from build123d import *

# Parameters (mm, degrees)
SKETCH1_W               = 78
SKETCH1_H               = 48
BOSS_EXTRUDE1_DEPTH     = 32
CUT_EXTRUDE1_DEPTH      = 1
CUT_EXTRUDE1_DEPTH_BACK = 49
SKETCH3_OUTSIDE_W       = 69.404
SKETCH3_OUTSIDE_H       = 53.404
CUT_EXTRUDE3_DEPTH      = 1
CUT_EXTRUDE3_DEPTH_BACK = 79
FILLET1_R               = 1.5
SKETCH4_R               = 4
CUT_EXTRUDE4_DEPTH      = 1
CUT_EXTRUDE4_DEPTH_BACK = 10
CHAMFER1_SIZE           = 1.5


with BuildPart() as part:
    # Sketch1 → Boss-Extrude1 (new body)
    with BuildSketch(Plane(origin=(0, 0, 0), x_dir=(1, 0, 0), z_dir=(0, 1, 0))):
        Rectangle(SKETCH1_W, SKETCH1_H)
    extrude(amount=BOSS_EXTRUDE1_DEPTH)

    # Sketch2 → Cut-Extrude1 (cut, two sides)
    with BuildSketch(Plane.XY.offset(24)) as cut_extrude1_sk:
        Polygon((-39, 13.33), (-35.438170518, 21.33), (-35.438170518, 32), (-39, 32), align=None)
        Polygon((35.438170518, 21.33), (35.438170518, 32), (39, 32), (39, 13.33), align=None)
    extrude(amount=CUT_EXTRUDE1_DEPTH, mode=Mode.SUBTRACT)
    extrude(cut_extrude1_sk.sketch, amount=-CUT_EXTRUDE1_DEPTH_BACK, mode=Mode.SUBTRACT)

    # Sketch3 outside → Cut-Extrude3 (cut, two sides)
    with BuildSketch(Plane(origin=(39, 0, 0), x_dir=(0, 0, -1), z_dir=(1, 0, 0))) as cut_extrude3_sk:
        with Locations((0, 16)):
            Rectangle(SKETCH3_OUTSIDE_W, SKETCH3_OUTSIDE_H)
        Polygon((-24, 8), (-18, 4.535898385), (-18, 32), (0, 32), (0, 25), (1.787630389, 26.5), (3.787630389, 26.5), (5.575260778, 25), (24, 25), (24, 10.67), (-4.8, 10.67), (-4.8, 0), (-24, 0), align=None, mode=Mode.SUBTRACT)
    extrude(amount=CUT_EXTRUDE3_DEPTH, mode=Mode.SUBTRACT)
    extrude(cut_extrude3_sk.sketch, amount=-CUT_EXTRUDE3_DEPTH_BACK, mode=Mode.SUBTRACT)

    # Fillet1
    fillet1_edges = [part.edges().sort_by_distance(p)[0] for p in [
        (0, 0, 24),
        (0, 10.67, 4.8),
        (0, 4.535898385, 18),
        (0, 0, 4.8),
        (0, 10.67, -24),
    ]]
    fillet(fillet1_edges, radius=FILLET1_R)

    # Sketch4 → Cut-Extrude4 (cut, two sides)
    with BuildSketch(Plane(origin=(0, 32, 0), x_dir=(1, 0, 0), z_dir=(0, 1, 0))) as cut_extrude4_sk:
        with Locations((0, -9)):
            Circle(SKETCH4_R)
        with Locations((23.438170518, -9)):
            Circle(SKETCH4_R)
        with Locations((-23.438170518, -9)):
            Circle(SKETCH4_R)
    extrude(amount=CUT_EXTRUDE4_DEPTH, mode=Mode.SUBTRACT)
    extrude(cut_extrude4_sk.sketch, amount=-CUT_EXTRUDE4_DEPTH_BACK, mode=Mode.SUBTRACT)

    # Chamfer1
    chamfer1_edges = [part.edges().sort_by_distance(p)[0] for p in [
        (-27.438170518, 32, 9),
        (19.438170518, 32, 9),
        (-4, 32, 9),
        (0, 25, -24),
    ]]
    chamfer(chamfer1_edges, length=CHAMFER1_SIZE)


solid = part.part
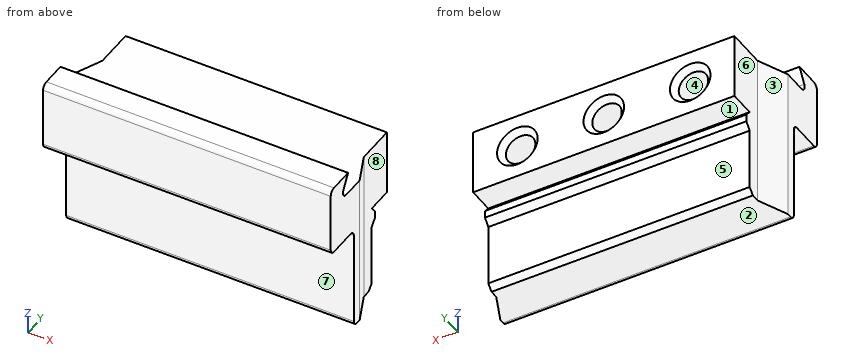
CAD build for the part. Positions are in the model's coordinates, mm. Face numbers are marked on the shaded views. A direction names the side the tool comes from. Give positions to 0.01 mm unless a question says otherwise; leave off trailing zeros. Loops run counter-clockwise (first coordinate to the right, second up) from the corner with the lowest first, then second, coordinate; pieces in that order, holes last. Notation, with made-up numbers: M -9,-23.75 L 23,-23.75 A27 cw 23,12.25 Z; hole C -23.5,4.25 d4. An arc over 180 degrees is marked long. One line per question, with ' | ' between items. Start each with the question number.
1. Saw through at D-D on z = -11. Give the cut face in (x, y), plus the area to 3 significant figures.
2. 3-axis set-ups, long thin cutter, end or side, ignore diameter. For the marked faces 4, 5, 6, 7 and 8: which of +Z, -Z, +X, -X, +Y, -Y reach the whole face in a straight line?
3. Two-plate mould, pull along Z, no slides. Class the marked faces 1, 2 and 3: pulls with the +Z half, pulls with the -Z half, needs draft (parallel to the pull), parting line crosses it, or undercut.
4. Flat gauge pins, fed straight in: pin 1 (6 mm diameter, centred on x = -14.5, y = 6, fed in from -Z); pin 2 (7.5 mm diameter, centred on x = -16, z = -7, fed in from -Y); pin 3 (5 mm diameter, centred on x = 16, z = -11, fed in from +Y). Where does each tip first touch, or does it go through?
5. Saw through at A-A on y = 28.5. Give the cut face in (x, z).
6. Saw through at B-B on x = 0. Give the cut face in (y, z), plus the area to 3 significant figures.
7. Probe L1, parallel to X at y = 25, z = 9; L2, parallel to Z at x = -15.5, y = 14; L3, parallel to Y at x = -30.5, z = 2. List the from-to ranges inside material, lowest first. Write a range as from..to.
8. Saw through at C-C on z = 9. Give the cut face in (x, y), plus the area to 3 significant figures.
Result sheet:
1) outline: M -39,10.67 L 39,10.67 L 39,13.33 L 35.44,21.33 L 35.44,25 L -35.44,25 L -35.44,21.33 L -39,13.33 Z | area: 1,060 mm^2
2) face 4: +Y | face 5: -Z, +X, -X, +Y | face 6: +Z, -Z, -X, +Y | face 7: -Z, +X, -X, -Y | face 8: +Z, -Z, +X, +Y
3) face 1: undercut | face 2: pulls with the -Z half | face 3: needs draft
4) pin 1: stops at z = 4.8 | pin 2: stops at y = 10.67 | pin 3: stops at y = 25
5) outline: M -35.44,0 L 35.44,0 L 35.44,18 L -35.44,18 Z; hole C -23.44,9 d8; hole C 0,9 d8; hole C 23.44,9 d8
6) outline: M 0,6.3 A1.5 ccw 1.5,4.8 L 9.17,4.8 A1.5 cw 10.67,3.3 L 10.67,-22.5 A1.5 ccw 12.17,-24 L 23.5,-24 L 25,-22.5 L 25,-5.58 L 26.5,-3.79 L 26.5,-1.79 L 25,0 L 32,0 L 32,3.5 L 30.5,5 L 22,5 L 22,13 L 30.5,13 L 32,14.5 L 32,18 L 7.13,18 A1.5 cw 5.83,20.25 L 8,24 L 1.5,24 A1.5 ccw 0,22.5 Z | area: 829 mm^2
7) L1: x = -35.44..-27.44, -19.44..-4, 4..19.44, 27.44..35.44 | L2: z = -24..18 | L3: y = 10.67..32
8) outline: M -39,0 L 39,0 L 39,13.33 L 35.44,21.33 L 35.44,32 L 28.94,32 L 27.44,30.5 L 27.44,22 L 19.44,22 L 19.44,30.5 L 17.94,32 L 5.5,32 L 4,30.5 L 4,22 L -4,22 L -4,30.5 L -5.5,32 L -17.94,32 L -19.44,30.5 L -19.44,22 L -27.44,22 L -27.44,30.5 L -28.94,32 L -35.44,32 L -35.44,21.33 L -39,13.33 Z | area: 2,140 mm^2
